Autodesk Inventor part; units mm, degrees
ref_plane "YZ Plane" through (0, 0, 0) normal (1, 0, 0) x (0, 1, 0)
ref_plane "XZ Plane" through (0, 0, 0) normal (0, 1, 0) x (-1, 0, 0)
ref_plane "XY Plane" through (0, 0, 0) normal (0, 0, 1) x (1, 0, 0)
sketch "Sketch1" plane through (0, 0, 0) normal (0, 0, 1) x (1, 0, 0)
  circle A0 centre (0, 0) radius 8
  circle A1 centre (0, 0) radius 2.5
  dimension "d0" = 16
  dimension "d1" = 5
extrude "Extrusion1" add sketch "Sketch1" along normal mid plane 5
sketch "Sketch2" plane through (0, 0, 2.5) normal (0, 0, 1) x (1, 0, 0)
  circle A0 centre (0, 0) radius 4.1451
  circle A1 centre (0, 0) radius 6.9091
extrude "Extrusion2" cut sketch "Sketch2" against normal blind 0.2
mirror "Mirror1" about plane through (0, 0, 0) normal (0, 0, 1) of "Extrusion2"
properties part number "625 Bearing"
Geometry check sheet. Reference: the model listing, model coordinates, mm. A direction names the side the tool comes from. Coordinates: 2 decimals unless noted, no trailing zeros. Order: outer loops, then holes, each group sorted by start corner. A loop starts at its lowest first (then second) coordinate and runs counter-clockwise, first axis right, second up. Notation, with made-up numbers: (-2, -18) - (5, -18) arc R13 cw to (5, -9) - close; hole circle Ø4 at (-15, -2). An arc over 180 degrees is marked (long way). Answer in a Markdown table with one row per item. Add a question column.
1) Cross-section at D-D, the plane y = 5.75. Record the cut outline in (x, z), then the cut area to 3 significant figures.
2) Cross-section at A-A, the plane y = 0. Record the cut outline in (x, z).
3) Cross-section at C-C, the plane z = -0.4. Record the cut outline in (x, y).
4) Material ranges on line 1 along Y through (x, z) = (0, -2.4); line 2 along Y through (x, z) = (0, 1.2); line 3 along Z through (x, y) = (5.5, -2), recorded low to high. Write a range as [from, to].
5) Release check for a two-part mould opening along X. For faces 3 (the cylindrical face through (-1.73, -7.81, 0.04)), 4 (the flat face through (-6, -4, -2.5)), 5 (the flat face through (0, -5, 2.3)) record: +X half, -X half, draft (parallel to the pull), parting line (faces both ways), or undercut.
6) Gauge pin test, flat ends, axial feed: P1, Ø2, axis at y = 1.5, z = 0.5, coming from the -X side; P2, Ø2, axis at x = -2.5, z = 0, coming from the +Y side; P3, Ø1.5, axis at x = -5.5, z = -2, coming from the -Y side. Record the tip position at first contact, or that the pin passes through.
7) Set-up check for faces 1 (the flat face through (0, -5, -2.3)), 2 (the cylindrical face through (-0.54, 2.44, -0.04)): record each of +Z, -Z, +X, -X, +Y, -Y from which the full face is reachable in a straight line by a thin tool's end or side.
Check result:
| question | item | result |
|---|---|---|
| 1 | outline | (-5.56, -2.5) - (-3.83, -2.5) - (-3.83, -2.3) - (3.83, -2.3) - (3.83, -2.5) - (5.56, -2.5) - (5.56, 2.5) - (3.83, 2.5) - (3.83, 2.3) - (-3.83, 2.3) - (-3.83, 2.5) - (-5.56, 2.5) - close |
| 1 | area | 52.6 mm² |
| 2 | outline | (-8, -2.5) - (-6.91, -2.5) - (-6.91, -2.3) - (-4.15, -2.3) - (-4.15, -2.5) - (-2.5, -2.5) - (-2.5, 2.5) - (-4.15, 2.5) - (-4.15, 2.3) - (-6.91, 2.3) - (-6.91, 2.5) - (-8, 2.5) - close; (2.5, -2.5) - (4.15, -2.5) - (4.15, -2.3) - (6.91, -2.3) - (6.91, -2.5) - (8, -2.5) - (8, 2.5) - (6.91, 2.5) - (6.91, 2.3) - (4.15, 2.3) - (4.15, 2.5) - (2.5, 2.5) - close |
| 3 | outline | circle Ø16 at (0, 0); hole circle Ø5 at (0, 0) |
| 4 | line 1 | y = [-8, -6.91], [-4.15, -2.5], [2.5, 4.15], [6.91, 8] |
| 4 | line 2 | y = [-8, -2.5], [2.5, 8] |
| 4 | line 3 | z = [-2.3, 2.3] |
| 5 | face 3 | parting line |
| 5 | face 4 | draft |
| 5 | face 5 | undercut |
| 6 | P1 | stops at x = -7.98 |
| 6 | P2 | stops at y = 7.86 |
| 6 | P3 | stops at y = -6.44 |
| 7 | face 1 | -Z |
| 7 | face 2 | +Z, -Z |
